The figure shows three views and two pictorial views of one solid part (mm, origin at its lowest corner). Answer the questions. Coordinates: 2 decimals unless noted, no trailing zeros. Write each loop counter-clockwise with the first axis right and the second up, starting at its lowest first coordinate (ties: lowest second). Pieces come first, ordered by that corner, then holes.
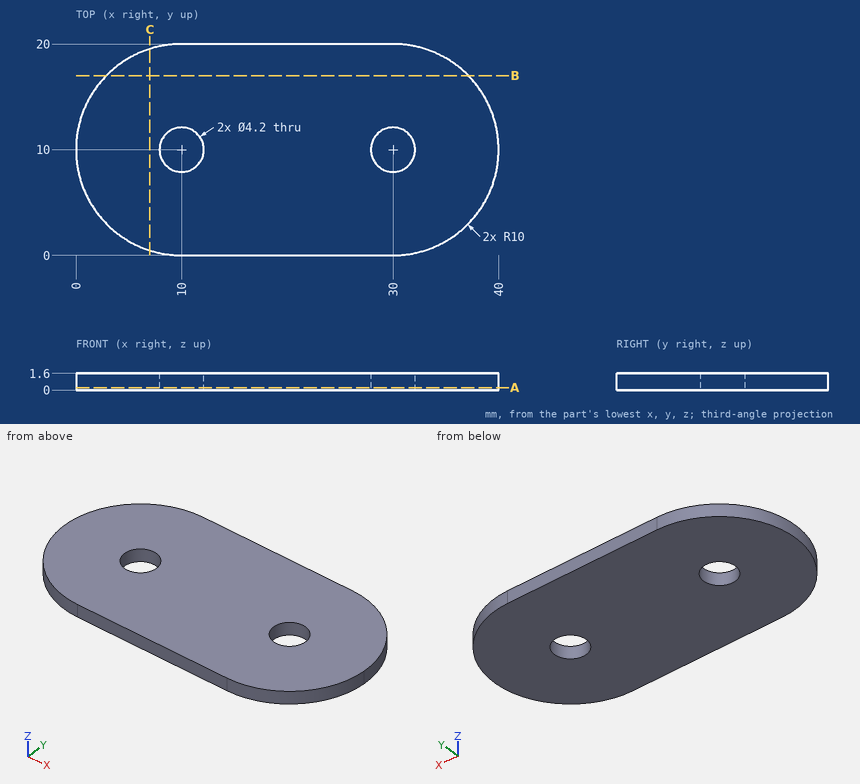
1. Section B-B on y = 17 is taken. Give the vertices of the cut face in (x, z), then the cut area to 3 significant figures.
Results found:
outline: (2.86, 0) - (37.14, 0) - (37.14, 1.6) - (2.86, 1.6) - close
area: 54.9 mm2
2. Section C-C on x = 7 is taken. Give the vertices of the cut face in (y, z).
Results found:
outline: (0.46, 0) - (19.54, 0) - (19.54, 1.6) - (0.46, 1.6) - close
3. Find the intervals of material crossed by L1, parallel to X at y = 8.5, z = 0.25; L2, parallel to Y at x = 30, z = 0.75; L3, parallel to Y at x = 31, z = 0.4, in increasing order.
Results found:
L1: x = 0.11 to 8.53, 11.47 to 28.53, 31.47 to 39.89
L2: y = 0 to 7.9, 12.1 to 20
L3: y = 0.05 to 8.15, 11.85 to 19.95
4. Section A-A on z = 0.25 is taken. Give the vertices of the cut face in (x, y), then the cut area to 3 significant figures.
Results found:
outline: (10, 0) - (30, 0) arc R10 ccw to (30, 20) - (10, 20) arc R10 ccw to start; hole circle Ø4.2 at (10, 10); hole circle Ø4.2 at (30, 10)
area: 686 mm2
